Part model, mm, in its own coordinate system. A direction names the side the tool comes from. Round coordinates to 2 decimals unless told otherwise and drop trailing zeros. Order: outer loops, then holes, each group sorted by start corner. A loop starts at its lowest first (then second) coordinate and runs counter-clockwise, first axis right, second up. Notation, with made-up numbers: (34.5, 79.25) - (73.5, 79.25) arc R21 ccw to (73.5, 105.25) - close; hole circle Ø4 at (33, -14). An arc over 180 degrees is marked (long way). Answer as a JSON object with one key per item and string values.
```python
from build123d import *

# Parameters (mm, degrees)
SKETCH1_R           = 80
BOSS_EXTRUDE1_DEPTH = 2.54
SKETCH2_R           = 75
SKETCH2_R_2         = 72.5
BOSS_EXTRUDE2_DEPTH = 25.4
SKETCH3_R           = 1.75
CUT_EXTRUDE1_DEPTH  = 116.953266448
SKETCH4_W           = 50.8
SKETCH4_H           = 25.4
CUT_EXTRUDE2_DEPTH  = 25.4
FILLET1_R           = 2.54


with BuildPart() as part:
    # Sketch1 → Boss-Extrude1 (new body)
    with BuildSketch(Plane(origin=(0, 0, 0), x_dir=(1, 0, 0), z_dir=(0, 1, 0))):
        with Locations(Location((0, 0, 0), (0, 0, 270))):
            Circle(SKETCH1_R)
    extrude(amount=BOSS_EXTRUDE1_DEPTH)

    # Sketch2 → Boss-Extrude2 (add)
    with BuildSketch(Plane(origin=(0, 2.54, 0), x_dir=(1, 0, 0), z_dir=(0, 1, 0))):
        with Locations(Location((0, 0, 0), (0, 0, 270))):
            Circle(SKETCH2_R)
        with Locations(Location((0, 0, 0), (0, 0, 270))):
            Circle(SKETCH2_R_2, mode=Mode.SUBTRACT)
    extrude(amount=BOSS_EXTRUDE2_DEPTH)

    # Sketch3 → Cut-Extrude1 (cut, through all)
    with BuildSketch(Plane(origin=(0, 2.54, 0), x_dir=(1, 0, 0), z_dir=(0, 1, 0))):
        with Locations(Location((0, 50, 0), (0, 0, 270))):
            Circle(SKETCH3_R)
        with Locations(Location((50, 0, 0), (0, 0, 270))):
            Circle(SKETCH3_R)
        with Locations(Location((0, -50, 0), (0, 0, 270))):
            Circle(SKETCH3_R)
        with Locations(Location((-50, 0, 0), (0, 0, 270))):
            Circle(SKETCH3_R)
        with Locations(Location((35.355339059, 35.355339059, 0), (0, 0, 270))):
            Circle(SKETCH3_R)
        with Locations(Location((35.355339059, -35.355339059, 0), (0, 0, 270))):
            Circle(SKETCH3_R)
        with Locations(Location((-35.355339059, -35.355339059, 0), (0, 0, 270))):
            Circle(SKETCH3_R)
        with Locations(Location((-35.355339059, 35.355339059, 0), (0, 0, 270))):
            Circle(SKETCH3_R)
        with Locations(Location((0, 0, 0), (0, 0, 270))):
            Circle(SKETCH3_R)
    extrude(amount=-CUT_EXTRUDE1_DEPTH, mode=Mode.SUBTRACT)

    # Sketch4 → Cut-Extrude2 (cut)
    with BuildSketch(Plane(origin=(0, 27.94, 0), x_dir=(1, 0, 0), z_dir=(0, 1, 0))):
        with Locations((0, -75)):
            Rectangle(SKETCH4_W, SKETCH4_H)
    extrude(amount=-CUT_EXTRUDE2_DEPTH, mode=Mode.SUBTRACT)

    # Fillet1
    fillet1_edges = [part.edges().sort_by_distance(p)[0] for p in [
        (0, 2.54, -72.5),
        (-25.4, 27.94, 69.236494294),
        (25.4, 27.94, 69.236494294),
        (-25.4, 2.54, 69.236494294),
        (25.4, 2.54, 69.236494294),
    ]]
    fillet(fillet1_edges, radius=FILLET1_R)


solid = part.part
```
Item 1: Drop flat-ended pins along their axis: P1, Ø8, axis at x = -7.5, z = -8, coming from the +Y side; P2, Ø10, axis at y = 8.5, z = -6.5, coming from the -X side (3 decimals); P3, Ø1.5, axis at x = 43.5, y = 10.5, coming from the +Z side; P4, Ø3, axis at x = 50, z = 0, coming from the -Y side. Give the stop position or say it passes through.
Taken from the geometry:
{"P1": "y = 2.54", "P2": "x = -74.985", "P3": "z = 61.62", "P4": "through"}
Item 2: Cut at A-A (y = 21.75). Write the cut outline in (x, z) (3 decimals).
Taken from the geometry:
{"outline": "(-25.4, 67.905) - (-25.4, 70.568) arc R75 ccw (long way) to (25.4, 70.568) - (25.4, 67.905) arc R72.5 cw (long way) to start"}
Item 3: Probe L1, parallel to X at y = 0.9, z = 0; L2, parallel to Y at x = 27, z = 11; L3, parallel to X at y = 0.95, z = 50. List the from-to ranges inside material, lowest first. Write a range as from..to.
Taken from the geometry:
{"L1": "-80..-51.75, -48.25..-1.75, 1.75..48.25, 51.75..80", "L2": "0..2.54", "L3": "-62.45..-1.75, 1.75..62.45"}
Item 4: Tool access for faces 1 (the cylindrical face through (-51.71, 1.29, -0.38)), 2 (the flat face through (1, 2.54, 17)): list every direction of +Z, -Z, +X, -X, +Y, -Y with a clear straight run to the whole face (end or side of a thin tool).
Taken from the geometry:
{"face 1": "+Y, -Y", "face 2": "+Y"}
Item 5: Two-plate mould, pull along X, no slides. Class faces 3 (the flat face through (6, 27.94, -73)), 4 (the cylindrical face through (34.29, 1.288, 33.967)), 5 (the cylindrical face through (2.97, 15.06, -74.94)): pulls with the +X half, pulls with the -X half, needs draft (parallel to the pull), parting line crosses it, or undercut.
Taken from the geometry:
{"face 3": "needs draft", "face 4": "undercut", "face 5": "parting line crosses it"}
